For this review, take the finished solid that the model builds, in its own axes (mm). Face numbers are marked on the shaded views. A direction names the side the tool comes from. Give positions to 0.01 mm unless a question says otherwise; leave off trailing zeros. Loops run counter-clockwise (first coordinate to the right, second up) from the corner with the lowest first, then second, coordinate; pieces in that order, holes last.
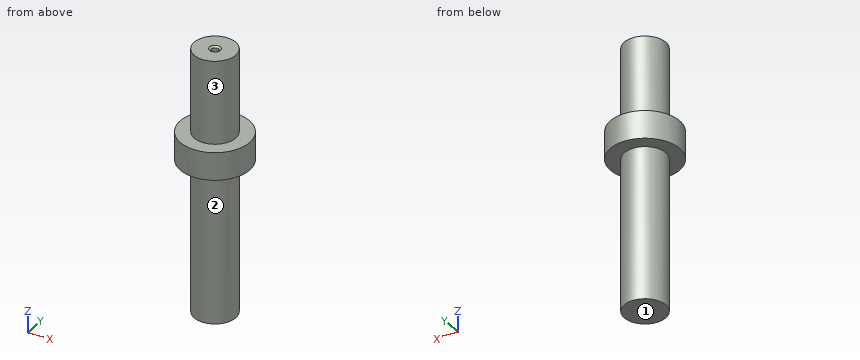
```python
from build123d import *

# Parameters (mm, degrees)
SKETCH1_R                       = 12.5
F_25MM_DIA_DEPTH                = 10
F_15MM_START                    = -10
SKETCH2_R                       = 7.5
F_15MM_DIA_BEARING_END_DEPTH    = 40
F_15MM_START_2                  = 55
SKETCH3_R                       = 7.5
F_15MM_DIA_GEAR_END_DEPTH       = 55
M3X0_5_TAPPED_HOLE1_D           = 2.5
M3X0_5_TAPPED_HOLE1_DEPTH       = 15
M3X0_5_TAPPED_HOLE1_CSINK_D     = 4
M3X0_5_TAPPED_HOLE1_CSINK_ANGLE = 120
M3X0_5_TAPPED_HOLE1_TIP         = 0.751075774


with BuildPart() as part:
    # Sketch1 → 25mm dia (new body)
    with BuildSketch(Plane.XY):
        Circle(SKETCH1_R)
    extrude(amount=F_25MM_DIA_DEPTH)

    # Sketch2 → 15mm dia bearing end (add)
    with BuildSketch(Plane.XY.offset(10).offset(F_15MM_START)):
        Circle(SKETCH2_R)
    extrude(amount=F_15MM_DIA_BEARING_END_DEPTH)

    # Sketch3 → 15mm dia gear end (add)
    with BuildSketch(Plane(origin=(0, 0, 0), x_dir=(-1, 0, 0), z_dir=(0, 0, -1)).offset(F_15MM_START_2)):
        with Locations(Location((0, 0, 0), (0, 0, 180))):
            Circle(SKETCH3_R)
    extrude(amount=-F_15MM_DIA_GEAR_END_DEPTH)

    # M3x0.5 Tapped Hole1
    with Locations(Plane.XY.offset(40)):
        with Locations((0, 0)):
            CounterSinkHole(M3X0_5_TAPPED_HOLE1_D / 2, M3X0_5_TAPPED_HOLE1_CSINK_D / 2, depth=M3X0_5_TAPPED_HOLE1_DEPTH, counter_sink_angle=M3X0_5_TAPPED_HOLE1_CSINK_ANGLE)
            with Locations((0, 0, -(M3X0_5_TAPPED_HOLE1_DEPTH + M3X0_5_TAPPED_HOLE1_TIP / 2))):  # 118° drill point
                Cone(0, M3X0_5_TAPPED_HOLE1_D / 2, M3X0_5_TAPPED_HOLE1_TIP, mode=Mode.SUBTRACT)


solid = part.part
```
Item 1: Take a section at A-A on y = -4.5. Give the boundary of the cut face in (x, z).
Answer:
outline: (-11.66, 0) - (-6, 0) - (-6, -55) - (6, -55) - (6, 0) - (11.66, 0) - (11.66, 10) - (6, 10) - (6, 40) - (-6, 40) - (-6, 10) - (-11.66, 10) - close
Item 2: Clearance check with flat-ended pins moving along their axes: pin 1 Ø2 at (x, z) = (3.5, -9) entering from -Y; pin 2 Ø8 at (y, z) = (4.5, 26.5) entering from +X; pin 3 Ø5 at (y, z) = (6, -40) entering from -X. State where each tip first meets the part, or that it passes through.
Answer:
pin 1: stops at y = -7.07
pin 2: stops at x = 7.48
pin 3: stops at x = -6.63
Item 3: Tool access review of the marked faces 1, 2 and 3: name each direction out of +Z, -Z, +X, -X, +Y, -Y from which nothing blocks a thin tool from reaching the whole face with its end or side.
Answer:
face 1: -Z, +X, -X, +Y, -Y
face 2: -Z
face 3: +Z
Item 4: Take a section at D-D on z = -31. Give the boundary of the cut face in (x, y).
Answer:
outline: circle Ø15 at (0, 0)
Item 5: For L1, parallel to X at y = 0, z = 32; L2, parallel to Z at x = 9.75, y = -0.75, list the stretches that pass through material, from the lowest coordinate up.
Answer:
L1: x = -7.5 to -1.25, 1.25 to 7.5
L2: z = 0 to 10
Item 6: Take a section at C-C on z = 29. Give the boundary of the cut face in (x, y).
Answer:
outline: circle Ø15 at (0, 0); hole circle Ø2.5 at (0, 0)
